Read the model definition and answer for the solid it produces. Units are mm, in the model's axes. Coordinates: 2 decimals unless noted, no trailing zeros. Order: outer loops, then holes, each group sorted by start corner. A loop starts at its lowest first (then second) coordinate and runs counter-clockwise, first axis right, second up.
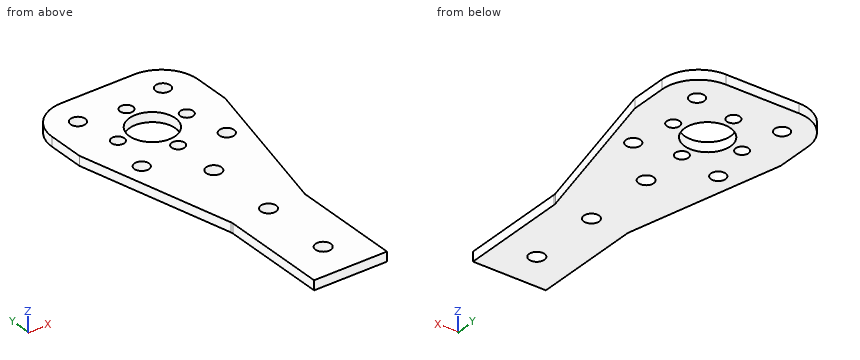
Autodesk Inventor part; units mm, degrees
ref_plane "YZ Plane" through (0, 0, 0) normal (1, 0, 0) x (0, 1, 0)
ref_plane "XZ Plane" through (0, 0, 0) normal (0, 1, 0) x (-1, 0, 0)
ref_plane "XY Plane" through (0, 0, 0) normal (0, 0, 1) x (1, 0, 0)
sketch "Sketch1" plane through (0, 0, 0) normal (0, 0, 1) x (1, 0, 0)
  circle A0 centre (22.225, 53.975) radius 8
  circle A1 centre (22.225, 25.4) radius 2.6543
  circle A2 centre (22.225, 0) radius 2.6543
  line L0 (9.525, 0) -> (34.925, 0)
  circle A3 centre (22.225, -25.4) radius 2.6604
  line L1 (34.925, 0) -> (34.925, -38.1)
  line L2 (34.925, -38.1) -> (9.525, -38.1)
  line L3 (9.525, -38.1) -> (9.525, 0)
  circle A4 centre (10.225, 53.975) radius 2.2479
  circle A5 centre (22.225, 65.975) radius 2.2479
  circle A6 centre (22.225, 41.975) radius 2.2479
  circle A7 centre (34.225, 53.975) radius 2.2479
  circle A8 centre (22.225, 53.975) radius 20.955 construction
  circle A9 centre (7.4168, 39.1484) radius 2.5527
  circle A10 centre (37.0516, 39.1668) radius 2.5527
  circle A11 centre (37.0332, 68.8016) radius 2.5527
  circle A12 centre (7.3984, 68.7832) radius 2.5527
  line L4 (-3.175, 79.375) -> (47.625, 79.375)
  line L5 (-3.175, 79.375) -> (-3.175, 53.975)
  line L6 (-3.175, 53.975) -> (9.525, 0)
  line L7 (47.625, 79.375) -> (47.625, 53.975)
  line L8 (47.625, 53.975) -> (34.925, 0)
  point P0 (0, 0)
  point P1 (0, 53.975)
  point P2 (44.45, 53.975)
  point P3 (22.225, 76.2)
  point P4 (24.8793, 0)
  point P5 (19.5707, 0)
  point P6 (22.225, 0)
  point P7 (22.225, 79.375)
  dimension "d36" = 41.91
  dimension "d2" = 16
  dimension "d3" = 5.3086
  dimension "d4" = 5.3086
  dimension "d5" = 22.225
  dimension "d26" = 25.4
  dimension "d27" = 38.1
  dimension "d28" = 25.4
  dimension "d29" = 28.575
  dimension "d30" = 53.975
  dimension "d31" = 4.4958
  dimension "d32" = 12
  dimension "d33" = 12
  dimension "d34" = 12
  dimension "d35" = 12
  dimension "d37" = 5.1054
  dimension "d38" = 14.8082
  dimension "d41" = 360
  dimension "d43" = 50.8
  dimension "d44" = 0
  dimension "d45" = 25.4
  dimension "d46" = 25.4
  dimension "d47" = 25.4
extrude "Extrusion1" add sketch "Sketch1" along normal blind 3.302 contours L0 L1 L2 L3 A2 | A2 L0 L6 L5 L4 L7 L8
fillet "Fillet13" radius 3.175 1 edges at (34.925, 0, 1.651)
fillet "Fillet14" radius 3.175 1 edges at (9.525, 0, 1.651)
fillet "Fillet15" radius 12.7 2 edges at (-3.175, 79.375, 1.651) (47.625, 79.375, 1.651)
properties part number "Arm Plate4"
1) A flat-ended cylindrical pin translates along its axis: pin 1 Ø1 at (y, z) = (-18.5, 1) entering from +X (3 decimals). Find the tip coordinate at first contact, or state that the pin passes through.
A:
pin 1: stops at x = 34.925
2) Straight lines are drawn through the part: line 1 (X direction, y = 54, z = 0.9) (3 decimals); line 2 (X direction, y = 70, z = 1.65); line 3 (X direction, y = 69.5, z = 0.25). For each, find the intervals that lie inside material, in ascending order.
A:
line 1: x = -3.175 to 7.977, 12.473 to 14.225, 30.225 to 31.977, 36.473 to 47.625
line 2: x = -2.73 to 5.15, 9.64 to 34.78, 39.29 to 47.18
line 3: x = -2.86 to 4.95, 9.85 to 34.58, 39.49 to 47.31
3) A cutting plane is placed at B-B, the plane z = 1.7. State how many separate pieces and enclosed holes the cut face has, and give its area (3 significant figures).
A:
separate pieces: 1
enclosed holes: 12
area: 3,830 mm2
4) A cutting plane is placed at A-A, the plane y = -25.4. Determine the outline of the cut face in (x, z) (3 decimals).
A:
outline: (9.525, 0) - (19.565, 0) - (19.565, 3.302) - (9.525, 3.302) - close; (24.885, 0) - (34.925, 0) - (34.925, 3.302) - (24.885, 3.302) - close
5) A cutting plane is placed at C-C, the plane x = 6.5. Determine the outline of the cut face in (y, z), and give its area (3 significant figures).
A:
outline: (12.86, 0) - (36.77, 0) - (36.77, 3.3) - (12.86, 3.3) - close; (41.53, 0) - (66.39, 0) - (66.39, 3.3) - (41.53, 3.3) - close; (71.17, 0) - (79.01, 0) - (79.01, 3.3) - (71.17, 3.3) - close
area: 187 mm2
6) A cutting plane is placed at D-D, the plane y = 25.4. Determine the outline of the cut face in (x, z), and give its area (3 significant figures).
A:
outline: (3.55, 0) - (19.57, 0) - (19.57, 3.3) - (3.55, 3.3) - close; (24.88, 0) - (40.9, 0) - (40.9, 3.3) - (24.88, 3.3) - close
area: 106 mm2
